Could you check a few things on this model? Use its own coordinates, in mm. A direction names the side the tool comes from. Coordinates: 2 decimals unless noted, no trailing zeros. Loops run counter-clockwise (first coordinate to the right, second up) from the corner with the lowest first, then second, coordinate; pieces in that order, holes last. Notation, with made-up numbers: M 75,-28 L 115,-28 A18 ccw 115,-22 Z; hole C -28,-27 d9. An arc over 180 degrees is marked long. Return JSON: item names as keys, results as strings. Group by question number.
Autodesk Inventor part; units mm, degrees
ref_plane "YZ Plane" through (0, 0, 0) normal (1, 0, 0) x (0, 1, 0)
ref_plane "XZ Plane" through (0, 0, 0) normal (0, 1, 0) x (-1, 0, 0)
ref_plane "XY Plane" through (0, 0, 0) normal (0, 0, 1) x (1, 0, 0)
sketch "main" plane through (0, 0, 0) normal (0, 0, 1) x (1, 0, 0)
  circle A0 centre (13.3958, 31.4064) radius 2.1844
  line L0 (25.3837, 29.1351) -> (22.5582, 29.1351)
  line L1 (25.3837, 29.1351) -> (25.3095, 29.1351)
  line L2 (20.0497, 41.8351) -> (13.668, 35.4534) construction
  arc A1 (20.0497, 41.8351) -> (15.6723, 40.0972) centre (20.0497, 35.4534) ccw
  circle A2 centre (25.3837, 35.4851) radius 2.1844
  line L3 (25.3837, 41.8351) -> (20.0497, 41.8351)
  line L4 (20.0497, 41.8351) -> (29.0749, 41.8351) construction
  arc A3 (25.3837, 29.1351) -> (25.3837, 41.8351) centre (25.3837, 35.4851) ccw
  circle A4 centre (12.6837, -15.3149) radius 2.1844
  circle A5 centre (-11.9225, -12.1399) radius 2.1844
  arc A6 (-16.0947, -14.4365) -> (-13.1988, -16.7282) centre (-11.9225, -12.1399) ccw
  line L5 (-9.1363, -0.7415) -> (-6.5789, -5.3874)
  line L6 (-22.634, -2.5568) -> (-16.0947, -14.4365)
  line L7 (-6.5789, -5.3874) -> (6.2826, -8.9649)
  line L8 (6.2826, -8.9649) -> (25.3837, -8.9649)
  circle A7 centre (25.3837, -15.3149) radius 2.1844
  arc A8 (25.3837, -21.6649) -> (25.3837, -8.9649) centre (25.3837, -15.3149) ccw
  line L9 (4.5492, -21.6649) -> (25.3837, -21.6649)
  line L10 (4.5492, -21.6649) -> (-13.1988, -16.7282)
  line L11 (22.5582, 29.1351) -> (-9.1363, -0.7415)
  line L12 (-21.4268, 5.126) -> (15.6723, 40.0972)
  circle A9 centre (-3.0276, 13.7434) radius 2.1844
  arc A10 (-21.4268, 5.126) -> (-22.634, -2.5568) centre (-17.0712, 0.5054) ccw
  point P0 (7.4272, 10.3782)
  point P1 (19.0337, 40.8191)
  point P2 (-25.006, 1.7522)
  point P3 (-30.1788, -11.3461)
  dimension "d0" = 4.3688
  dimension "d1" = 135
  dimension "d2" = 12.7
  dimension "d3" = 6.35
  dimension "d4" = 12.7
  dimension "d5" = 4.3688
  dimension "d6" = 4.3688
  dimension "d9" = 4.7625
  dimension "d10" = 47.625
  dimension "d11" = 37.3062
sketch "Sketch1" plane through (0, 0, 0) normal (0, 1, 0) x (-1, 0, 0)
  circle A0 centre (-4.0925, 11.9832) radius 2.1844
  line L0 (-6.35, -0.0073) -> (-6.3532, 2.8182)
  line L1 (-6.35, -0.0073) -> (-6.3501, 0.0669)
  line L2 (6.3439, 5.3413) -> (-0.0452, 11.7157) construction
  arc A1 (6.3439, 5.3413) -> (4.6009, 9.7167) centre (-0.0379, 5.334) ccw
  circle A2 centre (0, 0) radius 2.1844
  line L3 (6.35, 0.0073) -> (6.3439, 5.3413)
  line L4 (6.3439, 5.3413) -> (6.3542, -3.6839) construction
  arc A3 (-6.35, -0.0073) -> (6.35, 0.0073) centre (0, 0) ccw
  circle A4 centre (-50.8145, 12.6417) radius 2.1844
  circle A5 centre (-47.6678, 37.2516) radius 2.1844
  arc A6 (-49.9692, 41.4211) -> (-52.2575, 38.5226) centre (-47.6678, 37.2516) ccw
  line L5 (-36.2662, 34.4785) -> (-40.9092, 31.9157)
  line L6 (-38.097, 47.9741) -> (-49.9692, 41.4211)
  line L7 (-40.9092, 31.9157) -> (-44.4719, 19.0501)
  line L8 (-44.4719, 19.0501) -> (-44.45, -0.051)
  circle A7 centre (-50.8, -0.0583) radius 2.1844
  arc A8 (-57.15, -0.0656) -> (-44.45, -0.051) centre (-50.8, -0.0583) ccw
  line L9 (-57.1739, 20.769) -> (-57.15, -0.0656)
  line L10 (-57.1739, 20.769) -> (-52.2575, 38.5226)
  line L11 (-6.3532, 2.8182) -> (-36.2662, 34.4785)
  line L12 (-30.4128, 46.7757) -> (4.6009, 9.7167)
  circle A9 centre (-21.7743, 28.3864) radius 2.1844
  arc A10 (-30.4128, 46.7757) -> (-38.097, 47.9741) centre (-35.0285, 42.4147) ccw
  point P0 (0, 0)
  point P1 (-6.3501, 0.0669)
extrude "Extrusion1" add sketch "Sketch1" along normal blind 1.5875
properties part number "Ring Funnel" material "Acetal Resin, White"
(1) For faces 1 (the face through (-5.878, 0.783, 7.727)), 2 (the face through (38.555, 0.783, 33.215)), which set-ups out of +Z, -Z, +X, -X, +Y, -Y let a thin tool reach every point of the face, with its end or its side?
(2) Imagine slicing it at B-B, the plane z = 15.5. Write out the boundary of the cut face in (x, y).
(3) Imagine slicing it at D-D, the plane x = 50.8. Write out the boundary of the cut face in (y, z), then the cut area to 3 significant figures.
(4) If I drill on L1, parallel to Z at x = 50.8, y = 0.6; L2, parallel to X at y = 0.2, z = -2; L3, parallel to X at y = 1.3, z = 26.5, over which ranges is the centre line in solid material (lowest first)? Write a range as [from, to].
(5) We'd pull the mould along Z, two halves only. Please class faces 3 (the face through (26, 1.588, 28)), 4 (the face through (49.85, 0.78, 37.16)), 5 (the face through (21.1, 0.783, 18.427)), 6 (the face through (23.957, 0.783, 28.29)): +Z half, -Z half, draft (parallel to the pull), parting line (faces both ways), or undercut.
(6) Imagine slicing it at C-C, the plane y = 0.35. Write out the boundary of the cut face in (x, z).
(7) Imagine slicing it at A-A, the plane x = 1. Write out the boundary of the cut face in (y, z), then the cut area to 3 significant figures.
Checks:
{
 "1": {"face 1": "+Z, -X, +Y, -Y", "face 2": "-Z, +Y, -Y"},
 "2": {"outline": "M 0.86,0 L 18.34,0 L 18.34,1.59 L 0.86,1.59 Z; M 44.47,0 L 57.17,0 L 57.17,1.59 L 44.47,1.59 Z"},
 "3": {"outline": "M 0,-6.41 L 1.59,-6.41 L 1.59,-2.24 L 0,-2.24 Z; M 0,2.13 L 1.59,2.13 L 1.59,10.46 L 0,10.46 Z; M 0,14.83 L 1.59,14.83 L 1.59,40.84 L 0,40.84 Z", "area": "61.1 mm²"},
 "4": {"L1": "[-6.41, -2.24], [2.13, 10.46], [14.83, 40.84]", "L2": "[-6.03, -0.88], [0.88, 6.03], [44.75, 49.8], [51.8, 56.85]", "L3": "[11.26, 20.67], [22.88, 28.73], [42.41, 55.59]"},
 "5": {"face 3": "draft", "face 4": "undercut", "face 5": "-Z half", "face 6": "undercut"},
 "6": {"outline": "M -6.35,0.01 A6.35 ccw 6.35,-0.01 L 6.35,2.82 L 36.27,34.48 L 40.91,31.92 L 44.47,19.05 L 44.45,-0.05 A6.35 ccw 57.15,-0.07 L 57.17,20.77 L 52.26,38.52 A4.76 ccw 49.97,41.42 L 38.1,47.97 A6.35 ccw 30.41,46.78 L -4.6,9.72 A6.38 ccw -6.34,5.34 Z; hole C 0,0 d4.37; hole C 4.09,11.98 d4.37; hole C 21.77,28.39 d4.37; hole C 47.67,37.25 d4.37; hole C 50.8,-0.06 d4.37; hole C 50.81,12.64 d4.37"},
 "7": {"outline": "M 0,-6.27 L 1.59,-6.27 L 1.59,-1.94 L 0,-1.94 Z; M 0,1.94 L 1.59,1.94 L 1.59,15.64 L 0,15.64 Z", "area": "28.6 mm²"}
}
